Part model, mm, in its own coordinate system. A direction names the side the tool comes from. Coordinates: 2 decimals unless noted, no trailing zeros. Loops run counter-clockwise (first coordinate to the right, second up) from the corner with the lowest first, then second, coordinate; pieces in that order, holes last.
```python
from build123d import *

# Parameters (mm, degrees)
SKETCH_1_W                   = 42.3
SKETCH_1_H                   = 42.3
EXTRUDE_1_DEPTH              = 40
HOLE_WIZARD_M3_1_D           = 2.5
HOLE_WIZARD_M3_1_DEPTH       = 8.5
HOLE_WIZARD_M3_1_CSINK_D     = 3.05
HOLE_WIZARD_M3_1_CSINK_ANGLE = 90
HOLE_WIZARD_M3_1_TIP         = 0.751075774
SKETCH_6_R                   = 11
EXTRUDE_2_DEPTH              = 2
SKETCH_7_R                   = 2.5
CUT_EXTRUDE_1_DEPTH          = 54.203806255


with BuildPart() as part:
    # 스케치1 → 보스-돌출1 (new body)
    with BuildSketch(Plane.XY):
        Rectangle(SKETCH_1_W, SKETCH_1_H)
    extrude(amount=EXTRUDE_1_DEPTH)

    # M3 나사 구멍1
    with Locations(Plane.XY.offset(40)):
        with Locations((-15.5, 15.5), (15.5, 15.5), (15.5, -15.5), (-15.5, -15.5)):
            CounterSinkHole(HOLE_WIZARD_M3_1_D / 2, HOLE_WIZARD_M3_1_CSINK_D / 2, depth=HOLE_WIZARD_M3_1_DEPTH, counter_sink_angle=HOLE_WIZARD_M3_1_CSINK_ANGLE)
            with Locations((0, 0, -(HOLE_WIZARD_M3_1_DEPTH + HOLE_WIZARD_M3_1_TIP / 2))):  # 118° drill point
                Cone(0, HOLE_WIZARD_M3_1_D / 2, HOLE_WIZARD_M3_1_TIP, mode=Mode.SUBTRACT)

    # 스케치6 → 보스-돌출2 (add)
    with BuildSketch(Plane.XY.offset(40)):
        Circle(SKETCH_6_R)
    extrude_2 = extrude(amount=EXTRUDE_2_DEPTH)

    # 대칭 복사1: 보스-돌출2 across plane
    add(extrude_2.mirror(Plane(origin=(0, 0, 20), x_dir=(1, 0, 0), z_dir=(0, 0, -1))))

    # 스케치7 → 컷-돌출1 (cut, through all)
    with BuildSketch(Plane.XY.offset(42)):
        Circle(SKETCH_7_R)
    extrude(amount=-CUT_EXTRUDE_1_DEPTH, mode=Mode.SUBTRACT)


solid = part.part
```
Q1. Tool access for faces 1 (the flat face through (-3, 0, 42)), 2 (the cylindrical face through (-2.38, -10.74, -0.99)), 3 (the cylindrical face through (-14.579, 16.345, 35.555)): list every direction of +Z, -Z, +X, -X, +Y, -Y with a clear straight run to the whole face (end or side of a thin tool).
Q2. Probe line 1 (X direction, y = 15.5, z = 38.25); line 2 (X direction, y = -16, z = 38.5). List the from-to ranges inside material, lowest first.
Q3. Saw through at A-A (y = 0). List the corners of the cut face in (x, z).
Q4. Mould opens along Y. For faces 4 (the flat face through (0, 21.15, 20)), 5 (the cylindrical face through (-2.38, -10.74, 40.99)), 6 (the conical face through (-15.55, -15.71, 30.88)), 7 (the flat face through (-10, -9, 40)) say: released by +Y, released by -Y, zero draft, split by the parting line, or undercut.
Q5. Saw through at D-D (x = 8.5). List the corners of the cut face in (y, z).
Q6. Saw through at B-B (z = 37). List the corners of the cut face in (x, y), plus the area to 3 significant figures.
Q7. Drop flat-ended pins along their axis: P1, Ø5, axis at x = -14.5, y = -1.5, coming from the -Z side; P2, Ø3, axis at x = 15.5, y = 15.5, coming from the +Z side (3 decimals). Give the stop position or say it passes through.
Checked values:
1. face 1: +Z, +X, -X, +Y, -Y
1. face 2: -Z
1. face 3: +Z
2. line 1: x = -21.15 to -16.75, -14.25 to 14.25, 16.75 to 21.15
2. line 2: x = -21.15 to -16.65, -14.35 to 14.35, 16.65 to 21.15
3. outline: (-21.15, 0) - (-11, 0) - (-11, -2) - (-2.5, -2) - (-2.5, 42) - (-11, 42) - (-11, 40) - (-21.15, 40) - close; (2.5, -2) - (11, -2) - (11, 0) - (21.15, 0) - (21.15, 40) - (11, 40) - (11, 42) - (2.5, 42) - close
4. face 4: released by +Y
4. face 5: split by the parting line
4. face 6: undercut
4. face 7: zero draft
5. outline: (-21.15, 0) - (-6.98, 0) - (-6.98, -2) - (6.98, -2) - (6.98, 0) - (21.15, 0) - (21.15, 40) - (6.98, 40) - (6.98, 42) - (-6.98, 42) - (-6.98, 40) - (-21.15, 40) - close
6. outline: (-21.15, -21.15) - (21.15, -21.15) - (21.15, 21.15) - (-21.15, 21.15) - close; hole circle Ø2.5 at (-15.5, -15.5); hole circle Ø2.5 at (-15.5, 15.5); hole circle Ø5 at (0, 0); hole circle Ø2.5 at (15.5, -15.5); hole circle Ø2.5 at (15.5, 15.5)
6. area: 1,750 mm2
7. P1: stops at z = 0
7. P2: stops at z = 39.975
